Design review of the part built by this model. Coordinates are the model's own, in mm. A direction names the side the tool comes from. Coordinates: 2 decimals unless noted, no trailing zeros. Write each loop counter-clockwise with the first axis right and the second up, starting at its lowest first coordinate (ties: lowest second). Pieces come first, ordered by that corner, then holes. Notation, with made-up numbers: M 71,76 L 87,76 A32 cw 87,113 Z; hole C -26,68.25 d5. An arc over 180 degrees is marked long. One line per question, with ' | ' between items.
from build123d import *

# Parameters (mm, degrees)
SKETCH1_R            = 10
BOSS_EXTRUDE2_DEPTH  = 1
SKETCH3_R            = 5
BOSS_EXTRUDE3_DEPTH  = 14
CUT_EXTRUDE1_DEPTH   = 19
SKETCH5_R            = 12.5
BOSS_EXTRUDE4_DEPTH  = 1
CUT_EXTRUDE2_DEPTH   = 19
BOSS_EXTRUDE5_DEPTH  = 2
SKETCH8_R            = 7.5
BOSS_EXTRUDE6_DEPTH  = 2
SKETCH9_R            = 1
CUT_EXTRUDE3_DEPTH   = 25
CUT_EXTRUDE4_DEPTH   = 2
BOSS_EXTRUDE7_DEPTH  = 10
SKETCH14_R           = 1
CUT_EXTRUDE5_DEPTH   = 18
SKETCH15_R           = 1
BOSS_EXTRUDE8_DEPTH  = 17
SKETCH16_R           = 1
CUT_EXTRUDE7_DEPTH   = 10
CUT_EXTRUDE8_START   = -2
CUT_EXTRUDE8_DEPTH   = 2
SKETCH18_R           = 7.5
BOSS_EXTRUDE9_DEPTH  = 1.75
SKETCH19_R           = 7.5
SKETCH19_R_2         = 6.5
CUT_EXTRUDE9_DEPTH   = 1.75
BOSS_EXTRUDE11_START = -15
BOSS_EXTRUDE11_DEPTH = 15
SKETCH23_R           = 1
CUT_EXTRUDE10_DEPTH  = 8.75
SKETCH24_R           = 12.5
SKETCH24_R_2         = 7.5
CUT_EXTRUDE11_DEPTH  = 10
CUT_EXTRUDE12_START  = -10
SKETCH25_R           = 7.5
CUT_EXTRUDE12_DEPTH  = 10


with BuildPart() as part:
    # Sketch1 → Boss-Extrude2 (new body)
    with BuildSketch(Plane(origin=(0, 0, 0), x_dir=(1, 0, 0), z_dir=(0, 1, 0))):
        with Locations(Location((0, 0, 0), (0, 0, 270))):
            Circle(SKETCH1_R)
    extrude(amount=BOSS_EXTRUDE2_DEPTH)

    # Sketch3 → Boss-Extrude3 (add)
    with BuildSketch(Plane(origin=(0, 1, 0), x_dir=(1, 0, 0), z_dir=(0, 1, 0))):
        with Locations(Location((0, 0, 0), (0, 0, 270))):
            Circle(SKETCH3_R)
    extrude(amount=BOSS_EXTRUDE3_DEPTH)

    # Sketch4 → Cut-Extrude1 (cut)
    with BuildSketch(Plane(origin=(0, 15, 0), x_dir=(1, 0, 0), z_dir=(0, 1, 0))):
        with BuildLine():
            Line((0, -2), (0, 2))
            Line((0, 2), (-2.236067977, 2))
            ThreePointArc((-2.236067977, 2), (-3, 0), (-2.236067977, -2))
            Line((-2.236067977, -2), (0, -2))
        make_face()
        with BuildLine():
            Line((2.236067977, 2), (0, 2))
            Line((0, 2), (0, -2))
            Line((0, -2), (2.236067977, -2))
            ThreePointArc((2.236067977, -2), (2.802517077, -1.070466269), (3, 0))
            ThreePointArc((3, 0), (2.802517077, 1.070466269), (2.236067977, 2))
        make_face()
    extrude(amount=-CUT_EXTRUDE1_DEPTH, mode=Mode.SUBTRACT)

    # Sketch5 → Boss-Extrude4 (add)
    with BuildSketch(Plane(origin=(0, 1, 0), x_dir=(1, 0, 0), z_dir=(0, 1, 0))):
        with Locations(Location((0, 0, 0), (0, 0, 270))):
            Circle(SKETCH5_R)
    extrude(amount=-BOSS_EXTRUDE4_DEPTH)

    # Sketch6 → Cut-Extrude2 (cut)
    with BuildSketch(Plane(origin=(0, 1, 0), x_dir=(1, 0, 0), z_dir=(0, 1, 0))):
        with BuildLine():
            Line((2.236067977, 2), (-2.236067977, 2))
            ThreePointArc((-2.236067977, 2), (-3, 0), (-2.236067977, -2))
            Line((-2.236067977, -2), (2.236067977, -2))
            ThreePointArc((2.236067977, -2), (3, 0), (2.236067977, 2))
        make_face()
    extrude(amount=-CUT_EXTRUDE2_DEPTH, mode=Mode.SUBTRACT)

    # Sketch22 → Boss-Extrude11 (add)
    with BuildSketch(Plane.XZ.offset(BOSS_EXTRUDE11_START)):
        with BuildLine():
            Line((-2.236067977, 2), (2.236067977, 2))
            ThreePointArc((2.236067977, 2), (3, 0), (2.236067977, -2))
            Line((2.236067977, -2), (-2.236067977, -2))
            ThreePointArc((-2.236067977, -2), (-3, 0), (-2.236067977, 2))
        make_face()
        with BuildLine():
            ThreePointArc((2.167948339, -1.85), (2.85, 0), (2.167948339, 1.85))
            Line((2.167948339, 1.85), (-2.167948339, 1.85))
            ThreePointArc((-2.167948339, 1.85), (-2.85, 0), (-2.167948339, -1.85))
            Line((-2.167948339, -1.85), (2.167948339, -1.85))
        make_face(mode=Mode.SUBTRACT)
    extrude(amount=BOSS_EXTRUDE11_DEPTH)

    # Sketch24 → Cut-Extrude11 (cut)
    with BuildSketch(Plane(origin=(0, 1, 0), x_dir=(1, 0, 0), z_dir=(0, 1, 0))):
        Circle(SKETCH24_R)
        with Locations(Location((0, 0, 0), (0, 0, 270))):
            Circle(SKETCH24_R_2, mode=Mode.SUBTRACT)
    extrude(amount=-CUT_EXTRUDE11_DEPTH, mode=Mode.SUBTRACT)


with BuildPart() as body_2:
    # Sketch7 → Boss-Extrude5 (new body)
    with BuildSketch(Plane(origin=(0, 15, 0), x_dir=(1, 0, 0), z_dir=(0, 1, 0))):
        with BuildLine():
            Line((-2.236067977, -2), (2.236067977, -2))
            ThreePointArc((2.236067977, -2), (3, 0), (2.236067977, 2))
            Line((2.236067977, 2), (-2.236067977, 2))
            ThreePointArc((-2.236067977, 2), (-3, 0), (-2.236067977, -2))
        make_face()
    extrude(amount=BOSS_EXTRUDE5_DEPTH)

    # Sketch8 → Boss-Extrude6 (add)
    with BuildSketch(Plane(origin=(0, 17, 0), x_dir=(1, 0, 0), z_dir=(0, 1, 0))):
        with Locations(Location((0, 0, 0), (0, 0, 270))):
            Circle(SKETCH8_R)
    extrude(amount=BOSS_EXTRUDE6_DEPTH)

    # Sketch9 → Cut-Extrude3 (cut)
    with BuildSketch(Plane(origin=(0, 19, 0), x_dir=(1, 0, 0), z_dir=(0, 1, 0))):
        with Locations(Location((0, 0, 0), (0, 0, 270))):
            Circle(SKETCH9_R)
    extrude(amount=-CUT_EXTRUDE3_DEPTH, mode=Mode.SUBTRACT)

    # Sketch10 → Cut-Extrude4 (cut)
    with BuildSketch(Plane.XZ.offset(-15)):
        with BuildLine():
            Line((-2.121320344, -1.75), (2.121320344, -1.75))
            ThreePointArc((2.121320344, -1.75), (2.75, 0), (2.121320344, 1.75))
            Line((2.121320344, 1.75), (-2.121320344, 1.75))
            ThreePointArc((-2.121320344, 1.75), (-2.75, 0), (-2.121320344, -1.75))
        make_face()
    extrude(amount=-CUT_EXTRUDE4_DEPTH, mode=Mode.SUBTRACT)

    # Sketch11 → Boss-Extrude7 (add)
    with BuildSketch(Plane.XZ.offset(-17)):
        with BuildLine():
            Line((-2.121320344, -1.75), (2.121320344, -1.75))
            ThreePointArc((2.121320344, -1.75), (2.75, 0), (2.121320344, 1.75))
            Line((2.121320344, 1.75), (-2.121320344, 1.75))
            ThreePointArc((-2.121320344, 1.75), (-2.75, 0), (-2.121320344, -1.75))
        make_face()
    extrude(amount=BOSS_EXTRUDE7_DEPTH)

    # Sketch14 → Cut-Extrude5 (cut)
    with BuildSketch(Plane(origin=(0, 17, 0), x_dir=(1, 0, 0), z_dir=(0, 1, 0))):
        with Locations(Location((0, 0, 0), (0, 0, 270))):
            Circle(SKETCH14_R)
    extrude(amount=-CUT_EXTRUDE5_DEPTH, mode=Mode.SUBTRACT)

    # Sketch15 → Boss-Extrude8 (add)
    with BuildSketch(Plane.XZ.offset(-7)):
        with BuildLine():
            Line((-2.121320344, -1.75), (2.121320344, -1.75))
            ThreePointArc((2.121320344, -1.75), (2.75, 0), (2.121320344, 1.75))
            Line((2.121320344, 1.75), (-2.121320344, 1.75))
            ThreePointArc((-2.121320344, 1.75), (-2.75, 0), (-2.121320344, -1.75))
        make_face()
        with Locations(Location((0, 0, 0), (0, 0, 270))):
            Circle(SKETCH15_R, mode=Mode.SUBTRACT)
    extrude(amount=-BOSS_EXTRUDE8_DEPTH)

    # Sketch16 → Cut-Extrude7 (cut)
    with BuildSketch(Plane.XZ.offset(-7)):
        with BuildLine():
            Line((-2.121320344, -1.75), (2.121320344, -1.75))
            ThreePointArc((2.121320344, -1.75), (2.75, 0), (2.121320344, 1.75))
            Line((2.121320344, 1.75), (-2.121320344, 1.75))
            ThreePointArc((-2.121320344, 1.75), (-2.75, 0), (-2.121320344, -1.75))
        make_face()
        with Locations(Location((0, 0, 0), (0, 0, 90))):
            Circle(SKETCH16_R, mode=Mode.SUBTRACT)
    extrude(amount=-CUT_EXTRUDE7_DEPTH, mode=Mode.SUBTRACT)

    # Sketch17 → Cut-Extrude8 (cut)
    with BuildSketch(Plane.XZ.offset(-15).offset(CUT_EXTRUDE8_START)):
        with BuildLine():
            Line((-2.236067977, -2), (2.236067977, -2))
            ThreePointArc((2.236067977, -2), (3, 0), (2.236067977, 2))
            Line((2.236067977, 2), (-2.236067977, 2))
            ThreePointArc((-2.236067977, 2), (-3, 0), (-2.236067977, -2))
        make_face()
    extrude(amount=CUT_EXTRUDE8_DEPTH, mode=Mode.SUBTRACT)

    # Sketch18 → Boss-Extrude9 (add)
    with BuildSketch(Plane.XZ.offset(-17)):
        with Locations(Location((0, 0, 0), (0, 0, 270))):
            Circle(SKETCH18_R)
    extrude(amount=BOSS_EXTRUDE9_DEPTH)

    # Sketch19 → Cut-Extrude9 (cut)
    # profile 1 of 2: a face of its own
    with BuildSketch(Plane(origin=(0, 19, 0), x_dir=(1, 0, 0), z_dir=(0, 1, 0))):
        with Locations(Location((0, 0, 0), (0, 0, 90))):
            Circle(SKETCH19_R)
        Circle(SKETCH19_R_2, mode=Mode.SUBTRACT)
    # profile 2 of 2: a face of its own
    with BuildSketch(Plane(origin=(0, 19, 0), x_dir=(1, 0, 0), z_dir=(0, 1, 0))):
        Circle(SKETCH19_R_2)
        with BuildLine():
            Line((2.121320344, -1.75), (-2.121320344, -1.75))
            ThreePointArc((-2.121320344, -1.75), (-2.75, 0), (-2.121320344, 1.75))
            Line((-2.121320344, 1.75), (2.121320344, 1.75))
            ThreePointArc((2.121320344, 1.75), (2.75, 0), (2.121320344, -1.75))
        make_face(mode=Mode.SUBTRACT)
    extrude(amount=-CUT_EXTRUDE9_DEPTH, mode=Mode.SUBTRACT)

    # Sketch23 → Cut-Extrude10 (cut)
    with BuildSketch(Plane(origin=(0, 24, 0), x_dir=(1, 0, 0), z_dir=(0, 1, 0))):
        with Locations(Location((0, 0, 0), (0, 0, 90))):
            Circle(SKETCH23_R)
    extrude(amount=-CUT_EXTRUDE10_DEPTH, mode=Mode.SUBTRACT)

    # Sketch25 → Cut-Extrude12 (cut)
    with BuildSketch(Plane.XZ.offset(-15.25).offset(CUT_EXTRUDE12_START)):
        with Locations(Location((0, 0, 0), (0, 0, 90))):
            Circle(SKETCH25_R)
    extrude(amount=CUT_EXTRUDE12_DEPTH, mode=Mode.SUBTRACT)


solid = part.part
1. Draft analysis for pull direction Z (two halves, no side actions). For faces 4 (the face through (2.85, 7.6, -0.03)), 5 (the face through (0.1, 15, -2.2)), 6 (the face through (0.33, 0.507, -7.493)), state which applies: pulls with the +Z half, pulls with the -Z half, needs draft (parallel to the pull), parting line crosses it, or undercut.
Answer sheet:
face 4: undercut | face 5: needs draft | face 6: parting line crosses it
2. To check wall thickness, follow line 1 along Y through (x, z) = (4.75, -3); line 2 along Z through (x, y) = (1.75, 8.25); line 3 along X through (y, z) = (9, -0.75). State the ranges of each line that lie inside material, in increasing order. Write a range as [from, to].
Answer sheet:
line 1: [0, 1] | line 2: [-4.68, -1.85], [1.85, 4.68] | line 3: [-4.94, -2.75], [2.75, 4.94]
3. Take a section at A-A (z = 0). Write out the cut boundary in (x, y).
Answer sheet:
outline: M -7.5,0 L -2.85,0 L -2.85,15 L -5,15 L -5,1 L -7.5,1 Z; M 2.85,0 L 7.5,0 L 7.5,1 L 5,1 L 5,15 L 2.85,15 Z
4. Insertion check: pin 1 Ø6 at (y, z) = (7.5, -1.5) entering from +X; pin 2 Ø8 at (y, z) = (3.5, 4.5) entering from +X; pin 3 Ø6 at (x, y) = (3, 13) entering from -Z. Each pin has a flat end and moves straight along its axis. Give the tip position at first contact, or say it passes through.
Answer sheet:
pin 1: x = 5 | pin 2: x = 7.37 | pin 3: z = -5
5. Tool access review of faces 1 (the face through (0, 0, -3)), 2 (the face through (-2.85, 7.6, 0.03)), 3 (the face through (-2, 1, 5)): name each direction out of +Z, -Z, +X, -X, +Y, -Y from which nothing blocks a thin tool from reaching the whole face with its end or side.
Answer sheet:
face 1: +Z, -Z, +X, -X, -Y | face 2: +Y, -Y | face 3: +Y
6. Take a section at C-C (y = 13). Write out the cut boundary in (x, z).
Answer sheet:
outline: C 0,0 d10; hole M -2.17,-1.85 L 2.17,-1.85 A2.85 ccw 2.17,1.85 L -2.17,1.85 A2.85 ccw Z
7. Take a section at D-D (z = 6.5). Write out the cut boundary in (x, y).
Answer sheet:
outline: M -3.74,0 L 3.74,0 L 3.74,1 L -3.74,1 Z
8. Take a section at B-B (x = 0). Write out the cut boundary in (y, z), then the cut area to 3 significant figures.
Answer sheet:
outline: M 0,-7.5 L 1,-7.5 L 1,-5 L 15,-5 L 15,-1.85 L 0,-1.85 Z; M 0,1.85 L 15,1.85 L 15,5 L 1,5 L 1,7.5 L 0,7.5 Z | area: 99.5 mm^2
